from build123d import *

# Parameters (mm, degrees)
SKETCH1_W           = 161
SKETCH1_H           = 145
BOSS_EXTRUDE1_DEPTH = 3
BOSS_EXTRUDE2_DEPTH = 15
CUT_EXTRUDE1_DEPTH  = 3
CUT_EXTRUDE2_DEPTH  = 2
CUT_EXTRUDE3_DEPTH  = 12
CUT_EXTRUDE5_DEPTH  = 12
CUT_EXTRUDE6_DEPTH  = 20
CUT_EXTRUDE8_DEPTH  = 10
FILLET2_R           = 5
FILLET3_R           = 5
SKETCH11_R          = 1.5
SKETCH11_R_2        = 1.25
CUT_EXTRUDE9_DEPTH  = 10
SKETCH12_R          = 1.325
CUT_EXTRUDE10_DEPTH = 17
SKETCH13_R          = 3
CUT_EXTRUDE11_DEPTH = 8
SKETCH14_R          = 6.25
CUT_EXTRUDE12_DEPTH = 1
FILLET5_R           = 3
FILLET6_R           = 3


with BuildPart() as part:
    # Sketch1 → Boss-Extrude1 (new body)
    with BuildSketch(Plane(origin=(0, 0, 0), x_dir=(1, 0, 0), z_dir=(0, 1, 0))):
        with Locations((-80.5, 0)):
            Rectangle(SKETCH1_W, SKETCH1_H)
    extrude(amount=BOSS_EXTRUDE1_DEPTH)

    # Sketch2 → Boss-Extrude2 (add)
    with BuildSketch(Plane(origin=(0, 0, 0), x_dir=(1, 0, 0), z_dir=(0, 1, 0))):
        Polygon((0, 72.5), (0, 84.5), (-173, 84.5), (-173, -84.5), (0, -84.5), (0, -72.5), (-161, -72.5), (-161, 72.5), align=None)
    extrude(amount=BOSS_EXTRUDE2_DEPTH)

    # Sketch3 → Cut-Extrude1 (cut)
    with BuildSketch(Plane(origin=(0, 15, 0), x_dir=(1, 0, 0), z_dir=(0, 1, 0))):
        Polygon((-161, 44.1), (-161, 37.8), (-164.3, 37.8), (-164.3, 12.95), (-168.8, 12.95), (-168.8, 68.95), (-164.3, 68.95), (-164.3, 44.1), align=None)
        Polygon((-24.95, -75.8), (-49.8, -75.8), (-49.8, -72.5), (-56.1, -72.5), (-56.1, -75.8), (-80.95, -75.8), (-80.95, -80.3), (-24.95, -80.3), align=None)
        Polygon((-161, -38.5), (-161, -44.8), (-164.3, -44.8), (-164.3, -65.1), (-168.8, -65.1), (-168.8, -18.2), (-164.3, -18.2), (-164.3, -38.5), align=None)
        Polygon((-99.75, -80.3), (-99.75, -75.8), (-124.6, -75.8), (-124.6, -72.5), (-130.9, -72.5), (-130.9, -75.8), (-155.75, -75.8), (-155.75, -80.3), align=None)
        Polygon((-48.3, 75.8), (-48.3, 72.5), (-54.6, 72.5), (-54.6, 75.8), (-79.45, 75.8), (-79.45, 80.3), (-23.45, 80.3), (-23.45, 75.8), align=None)
    extrude(amount=-CUT_EXTRUDE1_DEPTH, mode=Mode.SUBTRACT)

    # Sketch4 → Cut-Extrude2 (cut)
    with BuildSketch(Plane(origin=(0, 12, 0), x_dir=(1, 0, 0), z_dir=(0, 1, 0))):
        Polygon((-54.6, 72.5), (-48.3, 72.5), (-48.3, 75.8), (-42.0875, 75.8), (-42.0875, 80.3), (-60.8125, 80.3), (-60.8125, 75.8), (-54.6, 75.8), align=None)
        Polygon((-161, 44.1), (-161, 37.8), (-164.3, 37.8), (-164.3, 27.850226284), (-168.8, 27.850226284), (-168.8, 50.3125), (-164.3, 50.3125), (-164.3, 44.1), align=None)
        Polygon((-168.8, -33.425), (-168.8, -49.875), (-164.3, -49.875), (-164.3, -44.8), (-161, -44.8), (-161, -38.5), (-164.3, -38.5), (-164.3, -33.425), align=None)
        Polygon((-130.9, -72.5), (-130.9, -75.8), (-137.1125, -75.8), (-137.1125, -80.3), (-118.3875, -80.3), (-118.3875, -75.8), (-124.6, -75.8), (-124.6, -72.5), align=None)
        Polygon((-56.1, -75.8), (-62.3125, -75.8), (-62.3125, -80.3), (-43.5875, -80.3), (-43.5875, -75.8), (-49.8, -75.8), (-49.8, -72.5), (-56.1, -72.5), align=None)
    extrude(amount=-CUT_EXTRUDE2_DEPTH, mode=Mode.SUBTRACT)

    # Sketch5 → Cut-Extrude3 (cut)
    with BuildSketch(Plane.ZY.offset(173)):
        with BuildLine():
            Line((-5.75, 10.5), (10.63, 10.5))
            ThreePointArc((10.63, 10.5), (13.63, 7.5), (10.63, 4.5))
            Line((10.63, 4.5), (-5.75, 4.5))
            ThreePointArc((-5.75, 4.5), (-8.75, 7.5), (-5.75, 10.5))
        make_face()
    extrude(amount=-CUT_EXTRUDE3_DEPTH, mode=Mode.SUBTRACT)

    # Sketch7 → Cut-Extrude5 (cut)
    with BuildSketch(Plane(origin=(0, 0, -84.5), x_dir=(-1, 0, 0), z_dir=(0, 0, -1))):
        with BuildLine():
            Line((-4.5375, 10.634328206), (11.8425, 10.634328206))
            ThreePointArc((11.8425, 10.634328206), (14.8425, 7.634328206), (11.8425, 4.634328206))
            Line((11.8425, 4.634328206), (-4.5375, 4.634328206))
            ThreePointArc((-4.5375, 4.634328206), (-7.5375, 7.634328206), (-4.5375, 10.634328206))
        make_face()
    extrude(amount=-CUT_EXTRUDE5_DEPTH, mode=Mode.SUBTRACT)

    # Sketch8 → Cut-Extrude6 (cut)
    with BuildSketch(Plane(origin=(0, 0, -84.5), x_dir=(-1, 0, 0), z_dir=(0, 0, -1))):
        with BuildLine():
            Line((142.36, 12.5), (151.36, 12.5))
            ThreePointArc((151.36, 12.5), (155.86, 8), (151.36, 3.5))
            Line((151.36, 3.5), (142.36, 3.5))
            ThreePointArc((142.36, 3.5), (137.86, 8), (142.36, 12.5))
        make_face()
    extrude(amount=-CUT_EXTRUDE6_DEPTH, mode=Mode.SUBTRACT)

    # Sketch10 → Cut-Extrude8 (cut)
    with BuildSketch(Plane(origin=(0, 0, 0), x_dir=(0, 0, -1), z_dir=(1, 0, 0))):
        Polygon((-80.5, 15), (-76.5, 15), (-76.5, 11), (-72.5, 11), (-72.5, 7), (-76.5, 7), (-76.5, 3), (-80.5, 3), (-80.5, 7), (-84.5, 7), (-84.5, 11), (-80.5, 11), align=None)
    extrude(amount=-CUT_EXTRUDE8_DEPTH, mode=Mode.SUBTRACT)

    # Fillet2
    fillet2_edges = [part.edges().sort_by_distance(p)[0] for p in [
        (-173, 7.5, 84.5),
    ]]
    fillet(fillet2_edges, radius=FILLET2_R)

    # Fillet3
    fillet3_edges = [part.edges().sort_by_distance(p)[0] for p in [
        (-173, 7.5, -84.5),
    ]]
    fillet(fillet3_edges, radius=FILLET3_R)

    # Sketch11 → Cut-Extrude9 (cut)
    with BuildSketch(Plane(origin=(0, 0, 0), x_dir=(0, 0, -1), z_dir=(1, 0, 0))):
        with Locations((78.5, 2.317164103)):
            Circle(SKETCH11_R)
        with Locations((78.5, 12.817164103)):
            Circle(SKETCH11_R_2)
    extrude(amount=-CUT_EXTRUDE9_DEPTH, mode=Mode.SUBTRACT)

    # Sketch12 → Cut-Extrude10 (cut)
    with BuildSketch(Plane(origin=(0, 0, 0), x_dir=(-1, 0, 0), z_dir=(0, -1, 0))):
        with Locations(Location((166.267766953, -77.767766953, 0), (0, 0, 90))):
            Circle(SKETCH12_R)
        with Locations(Location((90.35, -78.05, 0), (0, 0, 90))):
            Circle(SKETCH12_R)
        with Locations((-80.0525, -78.05)):
            Circle(SKETCH12_R)
        with Locations((-164.807766953, -77.767766953)):
            Circle(SKETCH12_R)
        with Locations((-164.807766953, 77.767766953)):
            Circle(SKETCH12_R)
        with Locations((-80.0525, 78.05)):
            Circle(SKETCH12_R)
        with Locations(Location((90.35, 77.767766953, 0), (0, 0, 90))):
            Circle(SKETCH12_R)
        with Locations(Location((166.267766953, 77.767766953, 0), (0, 0, 90))):
            Circle(SKETCH12_R)
    extrude(amount=-CUT_EXTRUDE10_DEPTH, mode=Mode.SUBTRACT)

    # Sketch13 → Cut-Extrude11 (cut)
    with BuildSketch(Plane.XZ):
        with Locations(Location((-166.267766953, -77.767766953, 0), (0, 0, 270))):
            Circle(SKETCH13_R)
        with Locations(Location((-90.35, -77.767766953, 0), (0, 0, 270))):
            Circle(SKETCH13_R)
        with Locations(Location((-166.267766953, 77.767766953, 0), (0, 0, 270))):
            Circle(SKETCH13_R)
        with Locations(Location((-90.35, 78.05, 0), (0, 0, 270))):
            Circle(SKETCH13_R)
    extrude(amount=-CUT_EXTRUDE11_DEPTH, mode=Mode.SUBTRACT)

    # Sketch14 → Cut-Extrude12 (cut)
    with BuildSketch(Plane(origin=(0, 0, 0), x_dir=(-1, 0, 0), z_dir=(0, -1, 0))):
        with Locations(Location((153, -64.5, 0), (0, 0, 90))):
            Circle(SKETCH14_R)
        with Locations(Location((153, 64.5, 0), (0, 0, 90))):
            Circle(SKETCH14_R)
    extrude(amount=-CUT_EXTRUDE12_DEPTH, mode=Mode.SUBTRACT)

    # Fillet5
    fillet5_edges = [part.edges().sort_by_distance(p)[0] for p in [
        (-164.3, 12.5, -44.1),
        (-164.3, 12.5, -37.8),
        (-56.1, 12.5, 75.8),
        (-49.8, 12.5, 75.8),
        (-164.3, 12.5, 38.5),
        (-164.3, 12.5, 44.8),
        (-130.9, 12.5, 75.8),
        (-124.6, 12.5, 75.8),
        (-48.3, 12.5, -75.8),
        (-54.6, 12.5, -75.8),
    ]]
    fillet(fillet5_edges, radius=FILLET5_R)

    # Fillet6
    # the kernel refuses this fillet: 3 mm, written as the material it adds along each edge
    with BuildSketch(Plane(origin=(-168.8, 15, -12.95), x_dir=(0, 0, -1), z_dir=(0, -1, 0)), Plane(origin=(-164.3, 15, -12.95), x_dir=(-1, 0, 0), z_dir=(0, -1, 0)), Plane(origin=(-164.3, 15, -68.95), x_dir=(0, 0, 1), z_dir=(0, -1, 0)), Plane(origin=(-168.8, 15, -68.95), x_dir=(1, 0, 0), z_dir=(0, -1, 0)), Plane(origin=(-168.8, 15, 18.2), x_dir=(1, 0, 0), z_dir=(0, -1, 0)), Plane(origin=(-164.3, 15, 18.2), x_dir=(0, 0, 1), z_dir=(0, -1, 0)), Plane(origin=(-168.8, 15, 65.1), x_dir=(0, 0, -1), z_dir=(0, -1, 0)), Plane(origin=(-164.3, 15, 65.1), x_dir=(-1, 0, 0), z_dir=(0, -1, 0)), Plane(origin=(-23.45, 15, -75.8), x_dir=(-1, 0, 0), z_dir=(0, -1, 0)), Plane(origin=(-23.45, 15, -80.3), x_dir=(0, 0, 1), z_dir=(0, -1, 0)), Plane(origin=(-79.45, 15, -75.8), x_dir=(0, 0, -1), z_dir=(0, -1, 0)), Plane(origin=(-79.45, 15, -80.3), x_dir=(1, 0, 0), z_dir=(0, -1, 0))) as fillet6_piece_1:
        with BuildLine():
            CenterArc((FILLET6_R, FILLET6_R), FILLET6_R, 180, 90)
            Line((0, FILLET6_R), (0, 0))
            Line((0, 0), (FILLET6_R, 0))
        make_face()
    extrude(amount=10.5)
    with BuildSketch(Plane(origin=(-155.75, 15, 75.8), x_dir=(0, 0, 1), z_dir=(0, -1, 0)), Plane(origin=(-155.75, 15, 80.3), x_dir=(1, 0, 0), z_dir=(0, -1, 0)), Plane(origin=(-99.75, 15, 80.3), x_dir=(0, 0, -1), z_dir=(0, -1, 0)), Plane(origin=(-99.75, 15, 75.8), x_dir=(-1, 0, 0), z_dir=(0, -1, 0)), Plane(origin=(-80.95, 15, 80.3), x_dir=(1, 0, 0), z_dir=(0, -1, 0)), Plane(origin=(-80.95, 15, 75.8), x_dir=(0, 0, 1), z_dir=(0, -1, 0)), Plane(origin=(-24.95, 15, 80.3), x_dir=(0, 0, -1), z_dir=(0, -1, 0)), Plane(origin=(-24.95, 15, 75.8), x_dir=(-1, 0, 0), z_dir=(0, -1, 0))) as fillet6_piece_2:
        with BuildLine():
            CenterArc((FILLET6_R, -FILLET6_R), FILLET6_R, 90, 90)
            Line((0, -FILLET6_R), (0, 0))
            Line((0, 0), (FILLET6_R, 0))
        make_face()
    extrude(amount=10.5)


solid = part.part
Can you work these out from the model? Positions are in its coordinate system, mm. A direction names the side the tool comes from. Give positions to 0.01 mm unless a question says otherwise; leave off trailing zeros. Order: outer loops, then holes, each group sorted by start corner. A loop starts at its lowest first (then second) coordinate and runs counter-clockwise, first axis right, second up. Notation, with made-up numbers: M 83.5,80.25 L 101.5,80.25 A19 ccw 101.5,89.25 Z; hole C -17.5,63.25 d2. An arc over 180 degrees is marked long. Use one line per item in the form item = value. Start each with the question number.
Item 1: If we section it at C-C (z = 25): Write out the boundary of the cut face in (x, y).
Item 2: Will these pins go through, and if not, where does the flat tip stop? pin 1 Ø12 at (x, z) = (-39.5, 65.5) entering from +Y; pin 2 Ø2.5 at (x, z) = (-166.27, -77.77) entering from +Y; pin 3 Ø11 at (x, z) = (-153, -64.5) entering from -Y.
Item 3: If I drill on line 1 along X through (y, z) = (13.5, 78.05) (3 decimals); line 2 along Z through (x, y) = (-116, 13.5); line 3 along Z through (x, y) = (-116, 5.75), over which ranges is the centre line in solid material (lowest first)?
Item 4: If we section it at B-B (z = -0.5): Write out the boundary of the cut face in (x, y), then the cut area to 3 significant figures.
Item 5: We'd pull the mould along Z, two halves only. Please class faces 1 (the flat face through (-5, 7, 82)), 2 (the flat face through (-82, 3, -1)), 3 (the flat face through (-82, 9, -72.5)), 4 (the cylindrical face through (-171.5, 7.6, 83.07)): +Z half, -Z half, draft (parallel to the pull), parting line (faces both ways), or undercut.
Item 6: If we section it at A-A (x = -19): Write out the boundary of the cut face in (y, z), then the cut area to 3 significant figures.
Item 7: For faces 5 (the flat face through (-92, 8, -78)), 6 (the flat face through (-6, 4.634, -79)), 7 (the flat face through (-52, 13, -80.3)), 8 (the flat face through (-167, 10.5, 2)), which set-ups out of +Z, -Z, +X, -X, +Y, -Y let a thin tool reach every point of the face, with its end or its side?
Outcome:
q1.outline = M -173,0 L 0,0 L 0,3 L -161,3 L -161,15 L -164.3,15 L -164.3,12 L -168.8,12 L -168.8,15 L -173,15 Z
q2.pin_1 = 3
q2.pin_2 = through
q2.pin_3 = 1
q3.line_1 = -173 to -167.562, -164.973 to -155.655, -99.845 to -91.675, -89.025 to -80.855, -25.045 to -10
q3.line_2 = -84.5 to -72.5, 72.5 to 75.8, 80.3 to 84.5
q3.line_3 = -84.5 to -72.5, 72.5 to 84.5
q4.outline = M -173,0 L 0,0 L 0,3 L -161,3 L -161,4.5 L -173,4.5 Z; M -173,10.5 L -161,10.5 L -161,15 L -173,15 Z
q4.area = 591 mm2
q5.face_1 = draft
q5.face_2 = undercut
q5.face_3 = undercut
q5.face_4 = +Z half
q6.outline = M 0,-84.5 L 15,-84.5 L 15,-72.5 L 3,-72.5 L 3,72.5 L 15,72.5 L 15,84.5 L 0,84.5 Z
q6.area = 795 mm2
q7.face_5 = -Y
q7.face_6 = -Z, +X
q7.face_7 = +Y
q7.face_8 = +X, -X
